Part model, mm, in its own coordinate system. A direction names the side the tool comes from. Give positions to 0.01 mm unless a question says otherwise; leave off trailing zeros. Write each loop counter-clockwise with the first axis right and the second up, starting at its lowest first coordinate (ties: lowest second). Pieces come first, ordered by that corner, then holes. Notation, with made-up numbers: M 55.25,-38.75 L 93.25,-38.75 A25 ccw 93.25,-13.75 Z; hole C 66,44 d6. An arc over 180 degrees is marked long. Use a Markdown table: item, result.
```python
from build123d import *

# Parameters (mm, degrees)
BOSS_EXTRUDE1_DEPTH     = 150
CUT_EXTRUDE1_DEPTH      = 112
CUT_EXTRUDE1_DEPTH_BACK = 112
CUT_EXTRUDE2_DEPTH      = 112
CUT_EXTRUDE2_DEPTH_BACK = 112
SKETCH5_R               = 28
CUT_EXTRUDE3_DEPTH      = 50
SKETCH6_R               = 31
CUT_EXTRUDE4_DEPTH      = 224


with BuildPart() as part:
    # Sketch1 → Boss-Extrude1 (new body)
    with BuildSketch(Plane(origin=(0, 0, 0), x_dir=(1, 0, 0), z_dir=(0, 1, 0))):
        Polygon((59.5, 0), (-59.5, 0), (-59.5, 150), (-81, 150), (-81, 212), (-112, 212), (-112, -45), (-50, -107), (50, -107), (112, -45), (112, 212), (81, 212), (81, 150), (59.5, 150), align=None)
    extrude(amount=BOSS_EXTRUDE1_DEPTH)

    # Sketch3 → Cut-Extrude1 (cut, two sides: drawn at the far end of the back side and taken through both)
    with BuildSketch(Plane(origin=(0, 0, 0), x_dir=(0, 0, -1), z_dir=(1, 0, 0)).offset(-CUT_EXTRUDE1_DEPTH_BACK)):
        Polygon((-107, 150), (-107, 114.20428331), (-45, 150), align=None)
        Polygon((-107, 0), (-45, 0), (-107, 35.79571669), align=None)
    extrude(amount=CUT_EXTRUDE1_DEPTH + CUT_EXTRUDE1_DEPTH_BACK, mode=Mode.SUBTRACT)

    # Sketch4 → Cut-Extrude2 (cut, two sides: drawn at the far end of the back side and taken through both)
    with BuildSketch(Plane(origin=(0, 0, 0), x_dir=(0, 0, -1), z_dir=(1, 0, 0)).offset(-CUT_EXTRUDE2_DEPTH_BACK)):
        with BuildLine():
            Line((212, 150), (88, 150))
            ThreePointArc((88, 150), (154.908396662, 132.868592609), (212, 94))
            Line((212, 94), (212, 150))
        make_face()
    extrude(amount=CUT_EXTRUDE2_DEPTH + CUT_EXTRUDE2_DEPTH_BACK, mode=Mode.SUBTRACT)

    # Sketch5 → Cut-Extrude3 (cut)
    with BuildSketch(Plane.XY.offset(107)):
        with Locations((0, 75)):
            Circle(SKETCH5_R)
    extrude(amount=-CUT_EXTRUDE3_DEPTH, mode=Mode.SUBTRACT)

    # Sketch6 → Cut-Extrude4 (cut)
    with BuildSketch(Plane(origin=(112, 0, 0), x_dir=(0, 0, -1), z_dir=(1, 0, 0))):
        with Locations((88, 75)):
            Circle(SKETCH6_R)
    extrude(amount=-CUT_EXTRUDE4_DEPTH, mode=Mode.SUBTRACT)


solid = part.part
```
1. Tool access for faces 1 (the flat face through (-112, 74, -56.7)), 2 (the flat face through (-70, 67, -150)): list every direction of +Z, -Z, +X, -X, +Y, -Y with a clear straight run to the whole face (end or side of a thin tool).
Findings below:
| item | result |
|---|---|
| face 1 | +Z, -Z, -X, +Y, -Y |
| face 2 | -Z, +Y, -Y |
2. Two-plate mould, pull along X, no slides. Class faces 3 (the flat face through (87, 74, 70)), 4 (the flat face through (-81, 74, 76)), 5 (the flat face through (0, 75, 57)), 6 (the flat face through (-2, 150, 7)): released by +X, released by -X, zero draft, split by the parting line, or undercut.
Findings below:
| item | result |
|---|---|
| face 3 | released by +X |
| face 4 | released by -X |
| face 5 | undercut |
| face 6 | zero draft |
3. Cut at B-B, the plane y = 75. Give the cut face in (x, z).
Findings below:
| item | result |
|---|---|
| outline | M -112,-212 L -81,-212 L -81,-150 L -59.5,-150 L -59.5,-119 L -112,-119 Z; M -112,-57 L -59.5,-57 L -59.5,0 L 59.5,0 L 59.5,-57 L 112,-57 L 112,45 L 50,107 L 28,107 L 28,57 L -28,57 L -28,107 L -50,107 L -112,45 Z; M 59.5,-150 L 81,-150 L 81,-212 L 112,-212 L 112,-119 L 59.5,-119 Z |
4. Drill centre lines: L1, parallel to X at y = 113.5, z = -15.5; L2, parallel to X at y = 60.5, z = -185; L3, parallel to Z at x = 35, y = 41. Where is each one in solid material? Low to high.
Findings below:
| item | result |
|---|---|
| L1 | -112 to -59.5, 59.5 to 112 |
| L2 | -112 to -81, 81 to 112 |
| L3 | 0 to 107 |
5. Cut at A-A, the plane z = -14.5. Give the cut face in (x, y).
Findings below:
| item | result |
|---|---|
| outline | M -112,0 L -59.5,0 L -59.5,150 L -112,150 Z; M 59.5,0 L 112,0 L 112,150 L 59.5,150 Z |
6. Cut at D-D, the plane x = -32.5. Give the cut face in (y, z).
Findings below:
| item | result |
|---|---|
| outline | M 0,0 L 150,0 L 150,45 L 114.2,107 L 35.8,107 L 0,45 Z |
7. Cut at C-C, the plane x = -91.5. Give the cut face in (y, z), then the cut area to 3 significant figures.
Findings below:
| item | result |
|---|---|
| outline | M 0,-212 L 94,-212 A200 ccw 150,-88 L 150,45 L 138.16,65.5 L 11.84,65.5 L 0,45 Z; hole C 75,-88 d62 |
| area | 36,000 mm2 |
8. Drop flat-ended pins along their axis: P1, Ø6.5, axis at x = 66.5, y = 54.5, coming from the -Z side; P2, Ø4, axis at x = -68, y = 38, coming from the +Z side. Give the stop position or say it passes through.
Findings below:
| item | result |
|---|---|
| P1 | z = -150 |
| P2 | z = 91 |
